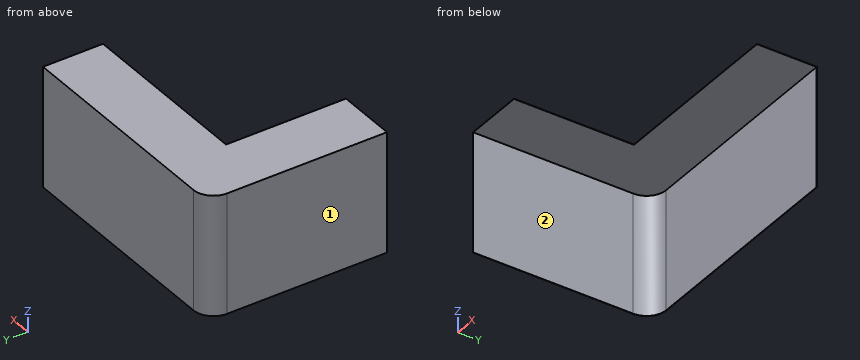
from build123d import *

# Parameters (mm, degrees)
F0_W     = 457.2
F0_H     = 914.4
F1_DEPTH = 914.4
F2_T     = -2.54


with BuildPart() as f1:
    # F0 (on Top) → F1 (new body)
    with BuildSketch(Plane.XY):
        with BuildLine():
            Line((682.751235, 631.639176), (-993.959226, 631.639176))
            ThreePointArc((-993.959226, 631.639176), (-1101.50277, 587.093182), (-1146.048765, 479.549638))
            Line((-1146.048765, 479.549638), (-1146.048765, 174.439176))
            Line((-1146.048765, 174.439176), (-688.848765, 174.439176))
            Line((-688.848765, 174.439176), (682.751235, 174.439176))
            Line((682.751235, 174.439176), (682.751235, 631.639176))
        make_face()
        with Locations((-917.448765, -282.760824)):
            Rectangle(F0_W, F0_H)
    extrude(amount=F1_DEPTH)

    # F2
    f2_openings = [f1.faces().sort_by_distance(p)[0] for p in [
        (-3.048765, 174.439176, 457.2),
        (682.751235, 403.039176, 457.2),
        (-917.448765, -739.960824, 457.2),
        (-688.848765, -282.760824, 457.2),
        (659.891235, 403.039176, 0),
    ]]
    offset(amount=F2_T, openings=f2_openings)


solid = f1.part
Geometry: final body of the model. Coordinates: model frame, mm. Face numbers are marked on the shaded views. A direction names the side the tool comes from. Coordinates: 2 decimals unless noted, no trailing zeros. Loops run counter-clockwise (first coordinate to the right, second up) from the corner with the lowest first, then second, coordinate; pieces in that order, holes last. Notation, with made-up numbers: (79.5, 18) - (119.5, 18) arc R15 ccw to (119.5, 38) - close; hole circle Ø10 at (63, 9.25). An arc over 180 degrees is marked (long way). Put each result on its own line as item: value. Start each with the question number.
Q1. Cut plane C-C, the plane y = -526.5. Return loops of the section in (x, z).
Q2. Line query: line 1 (X direction, y = -605.5, z = 566); line 2 (Y direction, x = 277, z = 614); line 3 (Z direction, x = -1048.5, y = -682). Output: solid intervals per line, ascending.
Q3. Set-up query: the marked faces 1 and 2. Return all of +Z, -Z, +X, -X, +Y, -Y with unobstructed straight access to the full face (end or side cutting, diameter ignored); none if empty.
Q4. Pin query (flat end, axial travel): pin 1 Ø5 at (x, y) = (-844.5, -248.5) entering from -Z; pin 2 Ø8 at (y, z) = (-23.5, 427) entering from +X; pin 3 Ø0.8 at (x, z) = (83, 913.5) entering from -Y. Return the tip coordinate at first contact, or that it passes through.
Q5. Cut plane B-B, the plane z = 437. Return loops of the section in (x, y).
Q6. Cut plane A-A, the plane x = 478.5. Return loops of the section in (y, z).
Filled sheet:
1. outline: (-1146.05, 0) - (-1143.51, 0) - (-1143.51, 911.86) - (-688.85, 911.86) - (-688.85, 914.4) - (-1146.05, 914.4) - close
2. line 1: -1146.05 to -1143.51
2. line 2: 629.1 to 631.64
2. line 3: 911.86 to 914.4
3. face 1: +Z, -Z, -X, +Y, -Y
3. face 2: -Z, +X, -Y
4. pin 1: z = 911.86
4. pin 2: x = -1143.51
4. pin 3: y = 174.44
5. outline: (-1146.05, -739.96) - (-1143.51, -739.96) - (-1143.51, 479.55) arc R149.55 cw to (-993.96, 629.1) - (682.75, 629.1) - (682.75, 631.64) - (-993.96, 631.64) arc R152.09 ccw to (-1146.05, 479.55) - close
6. outline: (174.44, 911.86) - (629.1, 911.86) - (629.1, 0) - (631.64, 0) - (631.64, 914.4) - (174.44, 914.4) - close
